Read the model definition and answer for the solid it produces. Units are mm, in the model's axes. Coordinates: 2 decimals unless noted, no trailing zeros. Use a Markdown table: item, result. Add a question column.
from build123d import *

# Parameters (mm, degrees)
SKETCH_1_W                  = 580
SKETCH_1_H                  = 285
EXTRUDE_1_DEPTH             = 10
HOLE_WIZARD_M5_1_AT_2_COUNT = 2
HOLE_WIZARD_M5_1_AT_2_PITCH = 50
HOLE_WIZARD_M5_1_AT_3_COUNT = 2
HOLE_WIZARD_M5_1_AT_3_PITCH = 100
HOLE_WIZARD_M5_1_AT_4_COUNT = 2
HOLE_WIZARD_M5_1_AT_4_PITCH = 150
HOLE_WIZARD_M5_1_AT_5_COUNT = 2
HOLE_WIZARD_M5_1_AT_5_PITCH = 200
HOLE_WIZARD_M5_1_AT_6_COUNT = 2
HOLE_WIZARD_M5_1_AT_6_PITCH = 250
HOLE_WIZARD_M5_2_D          = 4.2
HOLE_WIZARD_M5_3_D          = 4.2
SKETCH_12_R                 = 5
CUT_EXTRUDE_1_DEPTH         = 324.274264364
SKETCH_12_4_R               = 10
CUT_EXTRUDE_2_DEPTH         = 324.274264364


with BuildPart() as part:
    # 草图1 → 凸台-拉伸1 (new body)
    with BuildSketch(Plane.XY):
        Rectangle(SKETCH_1_W, SKETCH_1_H)
    extrude(amount=EXTRUDE_1_DEPTH)

    # 草图5 → M5 螺纹孔1 (revolve, cut)
    with BuildSketch(Plane(origin=(-290, 125, 5), x_dir=(0, 0, 1), z_dir=(0, 1, 0))):
        Polygon((0, 0), (0, 15.2618073), (2.1, 14), (2.1, 0), align=None)
    hole_wizard_m5_1 = revolve(axis=Axis((-296.35, 125, 5), (1, 0, 0)), mode=Mode.SUBTRACT)

    # M5 螺纹孔1 at 2: M5 螺纹孔1 ×2
    with Locations(*[(0, -i * HOLE_WIZARD_M5_1_AT_2_PITCH, 0) for i in range(1, HOLE_WIZARD_M5_1_AT_2_COUNT)]):
        add(hole_wizard_m5_1, mode=Mode.SUBTRACT)

    # M5 螺纹孔1 at 3: M5 螺纹孔1 ×2
    with Locations(*[(0, -i * HOLE_WIZARD_M5_1_AT_3_PITCH, 0) for i in range(1, HOLE_WIZARD_M5_1_AT_3_COUNT)]):
        add(hole_wizard_m5_1, mode=Mode.SUBTRACT)

    # M5 螺纹孔1 at 4: M5 螺纹孔1 ×2
    with Locations(*[(0, -i * HOLE_WIZARD_M5_1_AT_4_PITCH, 0) for i in range(1, HOLE_WIZARD_M5_1_AT_4_COUNT)]):
        add(hole_wizard_m5_1, mode=Mode.SUBTRACT)

    # M5 螺纹孔1 at 5: M5 螺纹孔1 ×2
    with Locations(*[(0, -i * HOLE_WIZARD_M5_1_AT_5_PITCH, 0) for i in range(1, HOLE_WIZARD_M5_1_AT_5_COUNT)]):
        add(hole_wizard_m5_1, mode=Mode.SUBTRACT)

    # M5 螺纹孔1 at 6: M5 螺纹孔1 ×2
    with Locations(*[(0, -i * HOLE_WIZARD_M5_1_AT_6_PITCH, 0) for i in range(1, HOLE_WIZARD_M5_1_AT_6_COUNT)]):
        add(hole_wizard_m5_1, mode=Mode.SUBTRACT)

    # 镜向1: M5 螺纹孔1 across plane
    add(hole_wizard_m5_1.mirror(Plane(origin=(0, 0, 0), x_dir=(0, 0, 1), z_dir=(1, 0, 0))), mode=Mode.SUBTRACT)

    # 镜向1 copy 1 sketch → 镜向1 copy 1 (revolve, cut)
    with BuildSketch(Plane(origin=(290, 75, 5), x_dir=(0, 0, 1), z_dir=(0, 1, 0))):
        Polygon((0, 0), (0, -15.2618073), (2.1, -14), (2.1, 0), align=None)
    revolve(axis=Axis((296.35, 75, 5), (1, 0, 0)), mode=Mode.SUBTRACT)

    # 镜向1 copy 2 sketch → 镜向1 copy 2 (revolve, cut)
    with BuildSketch(Plane(origin=(290, 25, 5), x_dir=(0, 0, 1), z_dir=(0, 1, 0))):
        Polygon((0, 0), (0, -15.2618073), (2.1, -14), (2.1, 0), align=None)
    revolve(axis=Axis((296.35, 25, 5), (1, 0, 0)), mode=Mode.SUBTRACT)

    # 镜向1 copy 3 sketch → 镜向1 copy 3 (revolve, cut)
    with BuildSketch(Plane(origin=(290, -25, 5), x_dir=(0, 0, 1), z_dir=(0, 1, 0))):
        Polygon((0, 0), (0, -15.2618073), (2.1, -14), (2.1, 0), align=None)
    revolve(axis=Axis((296.35, -25, 5), (1, 0, 0)), mode=Mode.SUBTRACT)

    # 镜向1 copy 4 sketch → 镜向1 copy 4 (revolve, cut)
    with BuildSketch(Plane(origin=(290, -75, 5), x_dir=(0, 0, 1), z_dir=(0, 1, 0))):
        Polygon((0, 0), (0, -15.2618073), (2.1, -14), (2.1, 0), align=None)
    revolve(axis=Axis((296.35, -75, 5), (1, 0, 0)), mode=Mode.SUBTRACT)

    # 镜向1 copy 5 sketch → 镜向1 copy 5 (revolve, cut)
    with BuildSketch(Plane(origin=(290, -125, 5), x_dir=(0, 0, 1), z_dir=(0, 1, 0))):
        Polygon((0, 0), (0, -15.2618073), (2.1, -14), (2.1, 0), align=None)
    revolve(axis=Axis((296.35, -125, 5), (1, 0, 0)), mode=Mode.SUBTRACT)

    # M5 螺纹孔2 (through all)
    with Locations(Plane(origin=(0, -142.5, 0), x_dir=(-1, 0, 0), z_dir=(0, -1, 0))):
        with Locations((0, -5), (-50, -5)):
            Hole(HOLE_WIZARD_M5_2_D / 2)

    # M5 螺纹孔3 (through all)
    with Locations(Plane.XY.offset(10)):
        with Locations((-160, -132.5), (-80, -132.5), (80, -132.5), (160, -132.5)):
            Hole(HOLE_WIZARD_M5_3_D / 2)

    # 草图12 → 切除-拉伸1 (cut, through all)
    with BuildSketch(Plane.XY.offset(10)):
        with Locations((-246, -55.15)):
            Circle(SKETCH_12_R)
        with Locations((-267.92, -77.07)):
            Circle(SKETCH_12_R)
        with Locations((-224.08, -77.07)):
            Circle(SKETCH_12_R)
    cut_extrude_1 = extrude(amount=-CUT_EXTRUDE_1_DEPTH, mode=Mode.SUBTRACT)

    # 镜向2: 切除-拉伸1 across plane
    add(cut_extrude_1.mirror(Plane(origin=(-2, 0, 0), x_dir=(0, 0, 1), z_dir=(1, 0, 0))), mode=Mode.SUBTRACT)

    # 草图12<4> → 切除-拉伸2 (cut, through all)
    with BuildSketch(Plane.XY.offset(10)):
        with Locations((-246, -77.5)):
            Circle(SKETCH_12_4_R)
    cut_extrude_2 = extrude(amount=-CUT_EXTRUDE_2_DEPTH, mode=Mode.SUBTRACT)

    # 镜向3: 切除-拉伸2 across plane
    add(cut_extrude_2.mirror(Plane(origin=(-2, 0, 0), x_dir=(0, 0, 1), z_dir=(1, 0, 0))), mode=Mode.SUBTRACT)


solid = part.part
Item 1: Consider probe 1 along Y at (x, z) = (-246, 4.25); probe 2 along Y at (x, z) = (80, 7.5); probe 3 along X at (y, z) = (48, 4.75). Determine where each line is inside the solid, lowest interval first.
Item 2: Determine the mould class of faces 1 (the cylindrical face through (-241.381, -57.065, 5.07)), 2 (the flat face through (290, -2, 5)), 3 (the flat face through (-4, -142.5, 5)) for opening direction Y: pulls with the +Y half, pulls with the -Y half, needs draft (parallel to the pull), parting line crosses it, or undercut.
Item 3: Each of these flat-tipped pins is pushed along its axis until it touches: pin 1 (4 mm diameter, centred on y = -25, z = 5, fed in from -X); pin 2 (8 mm diameter, centred on x = 220.08, y = -77.07, fed in from -Z); pin 3 (2.5 mm diameter, centred on y = 125, z = 5, fed in from -X); pin 4 (3.5 mm diameter, centred on y = -125, z = 5, fed in from +X). Where does it stop, or does it pass through?
Geometry says:
| question | item | result |
|---|---|---|
| 1 | probe 1 | y = -142.5 to -87.5, -67.5 to -60.15, -50.15 to 142.5 |
| 1 | probe 2 | y = -142.5 to -134.6, -130.4 to 142.5 |
| 1 | probe 3 | x = -290 to -2.09, 2.09 to 47.91, 52.09 to 290 |
| 2 | face 1 | undercut |
| 2 | face 2 | needs draft |
| 2 | face 3 | pulls with the -Y half |
| 3 | pin 1 | stops at x = -275.94 |
| 3 | pin 2 | passes through |
| 3 | pin 3 | stops at x = -275.49 |
| 3 | pin 4 | stops at x = 275.79 |
